```python
from build123d import *

# Parameters (mm, degrees)
F2_R     = 3.175
F3_DEPTH = 314.326
F4_SIZE  = 0.79375


with BuildPart() as f1:
    # F0 (on Front) → F1 (revolve)
    with BuildSketch(Plane.XZ):
        Polygon((0, 12.7), (0, 0), (314.325, 0), (314.325, 12.7), (198.4375, 12.7), (198.4375, 13.97), (179.3875, 13.97), (179.3875, 15.0114), (160.3375, 15.0114), (160.3375, 14.99997), (141.2875, 14.99997), (141.2875, 19.05), (131.7625, 19.05), (131.7625, 12.7), align=None)
    revolve(axis=Axis((157.1625, 0, 0), (1, 0, 0)))

    # F2 (on face) → F3 (cut, through all)
    with BuildSketch(Plane(origin=(0, 0, 0), x_dir=(0, -1, 0), z_dir=(-1, 0, 0))):
        Circle(F2_R)
    extrude(amount=-F3_DEPTH, mode=Mode.SUBTRACT)

    # F4
    f4_edges = [f1.edges().sort_by_distance(p)[0] for p in [
        (0, 0, -12.7),
        (314.325, 0, -12.7),
    ]]
    chamfer(f4_edges, length=F4_SIZE)


solid = f1.part
```
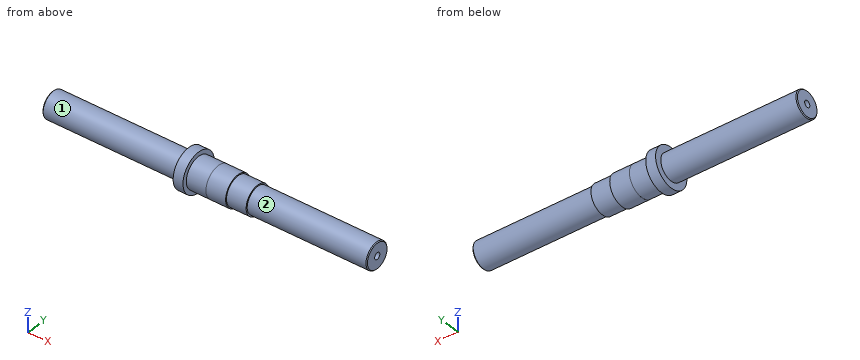
Here's how the part is built. I have some questions about the finished solid (model axes, mm). Face numbers are marked on the shaded views. A direction names the side the tool comes from. Give positions to 0.01 mm unless a question says otherwise; leave off trailing zeros. Loops run counter-clockwise (first coordinate to the right, second up) from the corner with the lowest first, then second, coordinate; pieces in that order, holes last. Notation, with made-up numbers: (-34.75, -4) -> (-9.75, -4) arc R25 cw to (-9.75, 33) -> close; hole circle Ø10 at (74.25, 74). An arc over 180 degrees is marked (long way). Use one line per item in the form item = value. Start each with the question number.
1) Please list where these lines run through material, in increasing order: line 1 along Z through (x, y) = (211, 0) (3 decimals); line 2 along Z through (x, y) = (170, 0) (3 decimals); line 3 along Y through (x, z) = (73.5, -1.5).
2) Imagine slicing it at C-C (x = 245). Please give me the cut outline in (y, z) (3 decimals).
3) Which directions (+Z, -Z, +X, -X, +Y, -Y) give clear straight access to the entire face, cutting with the end or side of a thin tool? Please do the marked faces 1 and 2.
4) For P1, Ø12, axis at x = 114.5, z = 14.5, coming from the -Y side; P2, Ø6, axis at x = 235.5, y = -8, coming from the +Z side; P3, Ø3, axis at x = 194, z = 1, coming from the +Y side; P4, Ø4, axis at y = 0, z = 0, coming from the -X side, each with a flat end and sliding along its axis, tell me the tip position at first contact or that it passes through.
5) Imagine slicing it at B-B (x = 172.5). Please give me the cut outline in (y, z) (3 decimals).
Check values:
q1.line_1 = -12.7 to -3.175, 3.175 to 12.7
q1.line_2 = -15.011 to -3.175, 3.175 to 15.011
q1.line_3 = -12.61 to -2.8, 2.8 to 12.61
q2.outline = circle Ø25.4 at (0, 0); hole circle Ø6.35 at (0, 0)
q3.face_1 = -X
q3.face_2 = +X
q4.P1 = -9.44
q4.P2 = 11.67
q4.P3 = 13.97
q4.P4 = through
q5.outline = circle Ø30.023 at (0, 0); hole circle Ø6.35 at (0, 0)
